Could you check a few things on this drawing? It's one solid part, dimensions in mm from its lowest x, y, z. A direction names the side the tool comes from. Coordinates: 2 decimals unless noted, no trailing zeros. Order: outer loops, then holes, each group sorted by start corner. A loop starts at its lowest first (then second) coordinate and runs counter-clockwise, first axis right, second up. Notation, with made-up numbers: (19.5, 34) - (32.5, 34) arc R17 ccw to (32.5, 47) - close; hole circle Ø9 at (30, -9). An arc over 180 degrees is marked (long way). Answer in a Markdown table with one row per item. Add a question column.
Item 1: I want a section at A-A (x = 4). Please give me the cut outline in (y, z), plus the area to 3 significant figures.
Item 2: I want a section at C-C (x = 23.5). Please give me the cut outline in (y, z), plus the area to 4 significant figures.
Item 3: If I drill on line 1 along Y through (x, z) = (3, 4.3); line 2 along Y through (x, z) = (6.5, 4.3); line 3 along Y through (x, z) = (17, 2.25), over which ranges is the centre line in solid material (lowest first)? Write a range as from..to.
Item 4: I want a section at B-B (z = 4.3). Please give me the cut outline in (x, y), plus the area to 3 significant figures.
Item 5: Will these pins go through, and if not, where does the flat tip stop? pin 1 Ø2.5 at (y, z) = (3.5, 2) entering from -X; pin 2 Ø1.5 at (x, z) = (30.5, 1.5) entering from -Y; pin 3 Ø2.5 at (y, z) = (67.5, 3.5) entering from -X; pin 4 Ø1.5 at (x, y) = (18, 33.5) entering from -Z.
Item 6: Thinking about a two-plate mould opening in Y: for the marked faces 4, 5 and 6, which applies, +Y half, -Y half, draft (parallel to the pull), parting line (faces both ways), or undercut?
Item 7: On a 3-axis mill with a long thin cutter (end or side, diameter ignored), from which of +Z, -Z, +X, -X, +Y, -Y can I reach the whole of each face in a straight line? I mean the marked faces 1, 2 and 3. Say none if no direction works.
Item 8: I want a section at D-D (y = 44). Please give me the cut outline in (x, z).
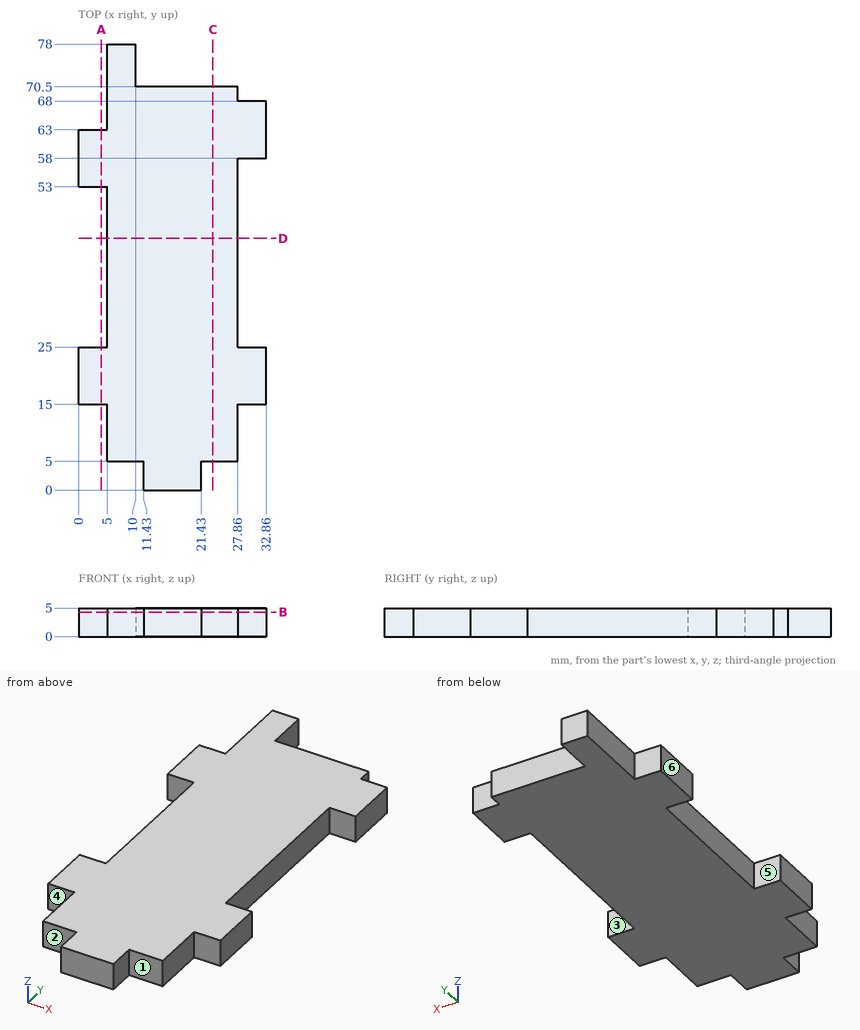
Values follow:
| question | item | result |
|---|---|---|
| 1 | outline | (15, 0) - (25, 0) - (25, 5) - (15, 5) - close; (53, 0) - (63, 0) - (63, 5) - (53, 5) - close |
| 1 | area | 100 mm^2 |
| 2 | outline | (5, 0) - (70.5, 0) - (70.5, 5) - (5, 5) - close |
| 2 | area | 327.5 mm^2 |
| 3 | line 1 | y = 15..25, 53..63 |
| 3 | line 2 | y = 5..78 |
| 3 | line 3 | y = 0..70.5 |
| 4 | outline | (0, 15) - (5, 15) - (5, 5) - (11.43, 5) - (11.43, 0) - (21.43, 0) - (21.43, 5) - (27.86, 5) - (27.86, 15) - (32.86, 15) - (32.86, 25) - (27.86, 25) - (27.86, 58) - (32.86, 58) - (32.86, 68) - (27.86, 68) - (27.86, 70.5) - (10, 70.5) - (10, 78) - (5, 78) - (5, 63) - (0, 63) - (0, 53) - (5, 53) - (5, 25) - (0, 25) - close |
| 4 | area | 1,780 mm^2 |
| 5 | pin 1 | stops at x = 11.43 |
| 5 | pin 2 | stops at y = 15 |
| 5 | pin 3 | stops at x = 5 |
| 5 | pin 4 | stops at z = 0 |
| 6 | face 4 | -Y half |
| 6 | face 5 | undercut |
| 6 | face 6 | draft |
| 7 | face 1 | +Z, -Z, +X, -Y |
| 7 | face 2 | +Z, -Z, -X, -Y |
| 7 | face 3 | +Z, -Z, +X |
| 8 | outline | (5, 0) - (27.86, 0) - (27.86, 5) - (5, 5) - close |
